Model file for the job. Use its own axes, mm. A direction names the side the tool comes from. Round coordinates to 2 decimals unless told otherwise and drop trailing zeros. Order: outer loops, then holes, each group sorted by start corner. A loop starts at its lowest first (then second) coordinate and runs counter-clockwise, first axis right, second up. Notation, with made-up numbers: (50, 7) -> (81, 7) arc R23 cw to (81, 24) -> close; hole circle Ø7 at (30, -34). An arc over 180 degrees is marked (long way). Put each result on its own line as item: value. Start each with the question number.
Q1. Probe L1, parallel to Y at x = -16.75, z = -68.5; L2, parallel to Z at x = -23.5, y = 28.6; L3, parallel to Z at x = -13.5, y = 23.5. List the from-to ranges inside material, lowest first.
Q2. Cut at C-C, the plane x = -27.25. List the corners of the cut face in (y, z), and give its area (3 significant figures).
Q3. Cut at D-D, the plane z = -9. List the corners of the cut face in (x, y).
Q4. Cut at A-A, the plane x = -6.5. List the corners of the cut face in (y, z).
Q5. Flat gauge pins, fed straight in: P1, Ø12, axis at y = 6.5, z = -33, coming from the -X side; P2, Ø6, axis at x = -23.5, z = -37.03, coming from the -Y side; P3, Ø10, axis at x = -25.5, y = 23, coming from the +Z side; P4, Ø9.5, axis at x = -11, z = -60, coming from the +Y side. Where does each tip first touch, or does it go through?
Q6. Cut at B-B, the plane y = 13. List the corners of the cut face in (x, z), and give its area (3 significant figures).
Q7. 3-axis set-ups, long thin cutter, end or side, ignore diameter. For faces 4 (the face through (-15.21, 14.676, -23.932)), 5 (the face through (-15, 0.76, -9)), 6 (the face through (-15, 0.76, -65)), 7 (the face through (-30, 13, -23)), 8 (the face through (-15, 29.174, -37)): which of +Z, -Z, +X, -X, +Y, -Y reach the whole face in a straight line?
Q8. Pull direction X, two halves, no side cores. Call faces 1 (the face through (-7.04, 28.8, -34.59)), 2 (the face through (0, 13, -23)), 3 (the face through (-14.79, 28.85, -46.8)): released by +X, released by -X, zero draft, split by the parting line, or undercut.
Autodesk Inventor part; units mm, degrees
ref_plane "YZ Plane" through (0, 0, 0) normal (1, 0, 0) x (0, 1, 0)
ref_plane "XZ Plane" through (0, 0, 0) normal (0, 1, 0) x (-1, 0, 0)
ref_plane "XY Plane" through (0, 0, 0) normal (0, 0, 1) x (1, 0, 0)
sketch "Boceto1" plane through (0, 0, 0) normal (0, 1, 0) x (-1, 0, 0)
  point P0 (0, 0)
sketch "Boceto2" plane through (0, 0, 0) normal (0, 1, 0) x (-1, 0, 0)
  line L0 (0, 0) -> (30, 0)
  line L1 (30, 0) -> (30, -20)
  line L2 (30, -20) -> (0, -20)
  line L3 (0, -20) -> (0, 0)
  dimension "d0" = 30
  dimension "d1" = 20
extrude "Placa1" add sketch "Boceto2" along normal blind 0.76
sketch "Boceto3" plane through (0, 0.1967, -19.2659) normal (0, -0.258819, -0.9659258) x (-1, 0, 0)
  line L0 (30, 0) -> (0, 0)
  line L1 (0, 0) -> (0, -30)
  line L2 (0, -30) -> (30, -30)
  line L3 (30, -30) -> (30, 0)
edge flange "Pestaña1" height 30 angle -75 thickness 0.76 bend radius 0.76 thickness toward (0, -0.258819, -0.9659258) relief tear relief width 0.76 relief depth 0.38 edges at (-15, 0, -20) wall of the first edge with corners at (-30, 0.1967, -19.2659) (0, 0.1967, -19.2659) (0, 29.1745, -27.0305) (-30, 29.1745, -27.0305)
bend "Doblez1"
corner "Esquina1"
sketch "Boceto4" plane through (-30, 28.4145, -27.0305) normal (0, 1, 0) x (-1, 0, 0)
  line L0 (-30, 0) -> (0, 0)
  line L1 (0, 0) -> (0, 20)
  line L2 (0, 20) -> (-30, 20)
  line L3 (-30, 20) -> (-30, 0)
edge flange "Pestaña2" height 20 angle -75 thickness 0.76 bend radius 0.76 thickness toward (0, 1, 0) relief tear relief width 0.76 relief depth 0.38 edges at (-15, 29.1745, -27.0305) wall of the first edge with corners at (0, 28.4145, -27.0305) (-30, 28.4145, -27.0305) (-30, 28.4145, -47.0305) (0, 28.4145, -47.0305)
bend "Doblez2"
corner "Esquina2"
sketch "Boceto5" plane through (-30, 28.9778, -46.2964) normal (0, 0.258819, -0.9659258) x (1, 0, 0)
  line L0 (30, 0) -> (0, 0)
  line L1 (0, 0) -> (0, -30)
  line L2 (0, -30) -> (30, -30)
  line L3 (30, -30) -> (30, 0)
edge flange "Pestaña3" height 30 angle -75 thickness 0.76 bend radius 0.76 thickness toward (0, 0.258819, -0.9659258) relief tear relief width 0.76 relief depth 0.38 edges at (-15, 29.1745, -47.0305) wall of the first edge with corners at (0, 28.9778, -46.2964) (-30, 28.9778, -46.2964) (-30, 0, -54.0609) (0, 0, -54.0609)
bend "Doblez3"
corner "Esquina3"
sketch "Boceto6" plane through (0, 0.76, -54.0609) normal (0, -1, 0) x (1, 0, 0)
  line L0 (-30, 0) -> (0, 0)
  line L1 (0, 0) -> (0, 20)
  line L2 (0, 20) -> (-30, 20)
  line L3 (-30, 20) -> (-30, 0)
edge flange "Pestaña4" height 20 angle -75 thickness 0.76 bend radius 0.76 thickness toward (0, -1, 0) relief tear relief width 0.76 relief depth 0.38 edges at (-15, 0, -54.0609) wall of the first edge with corners at (-30, 0.76, -54.0609) (0, 0.76, -54.0609) (0, 0.76, -74.0609) (-30, 0.76, -74.0609)
bend "Doblez4"
corner "Esquina4"
sketch "Boceto7" plane through (-30, 29.1745, -28.1968) normal (0, 1, 0) x (1, 0, 0)
  circle A0 centre (6.5, 8.8337) radius 2.5
  circle A1 centre (23.5, 8.8337) radius 2.5
  line L0 (0, 0) -> (0, 17.6673)
  line L1 (30, 0) -> (30, 17.6673)
  point P0 (30, -28.1968)
  dimension "d43" = 5
  dimension "d44" = 5
  dimension "d45" = 6.5
  dimension "d46" = 6.5
extrude "Extrusión1" cut sketch "Boceto7" against normal through all
equation "\"d46\" = d45"
equation "\"d2\" = Grosor"
equation "\"d3\" = Anchura_desahogo_plegado"
equation "\"d4\" = Profundidad_desahogo_plegado"
equation "\"d5\" = Remanente_mínimo"
equation "\"d6\" = Radiodetransición"
equation "\"d9\" = Radio_pliegue"
equation "\"d10\" = Tamaño_destalonado"
equation "\"d11\" = TamañoSeparación"
equation "\"d12\" = Tamaño_de_radio_de_Jacobi"
equation "\"d13\" = Anchura_desahogo_plegado"
equation "\"d14\" = Profundidad_desahogo_plegado"
equation "\"d15\" = Remanente_mínimo"
equation "\"d16\" = Radiodetransición"
equation "\"d19\" = Radio_pliegue"
equation "\"d20\" = Tamaño_destalonado"
equation "\"d21\" = TamañoSeparación"
equation "\"d22\" = Tamaño_de_radio_de_Jacobi"
equation "\"d23\" = Anchura_desahogo_plegado"
equation "\"d24\" = Profundidad_desahogo_plegado"
equation "\"d25\" = Remanente_mínimo"
equation "\"d26\" = Radiodetransición"
equation "\"d29\" = Radio_pliegue"
equation "\"d30\" = Tamaño_destalonado"
equation "\"d31\" = TamañoSeparación"
equation "\"d32\" = Tamaño_de_radio_de_Jacobi"
equation "\"d33\" = Anchura_desahogo_plegado"
equation "\"d34\" = Profundidad_desahogo_plegado"
equation "\"d35\" = Remanente_mínimo"
equation "\"d36\" = Radiodetransición"
equation "\"d39\" = Radio_pliegue"
equation "\"d40\" = Tamaño_destalonado"
equation "\"d41\" = TamañoSeparación"
equation "\"d42\" = Tamaño_de_radio_de_Jacobi"
equation "\"Radio_pliegue\" = Grosor"
equation "\"Anchura_desahogo_plegado\" = Grosor"
equation "\"Profundidad_desahogo_plegado\" = 0.5 * Grosor"
equation "\"Tamaño_destalonado\" = 4 * Grosor"
equation "\"Remanente_mínimo\" = 2 * Grosor"
equation "\"Radiodetransición\" = Radio_pliegue"
equation "\"Tamaño_de_radio_de_Jacobi\" = Radio_pliegue"
equation "\"TamañoSeparación\" = Grosor"
properties part number "placa tierra" material "Acero AISI 1006 85 LC"
Ans:
1. L1: y = 0 to 0.76
1. L2: z = -47.05 to -39.53, -34.53 to -27.01
1. L3: z = -48.55 to -47.76, -26.3 to -25.51
2. outline: (0, -74.06) -> (0.76, -74.06) -> (0.76, -55.23) arc R0.76 cw to (1.32, -54.49) -> (28.05, -47.33) arc R1.52 ccw to (29.17, -45.86) -> (29.17, -28.2) arc R1.52 ccw to (28.05, -26.73) -> (1.32, -19.57) arc R0.76 cw to (0.76, -18.83) -> (0.76, 0) -> (0, 0) -> (0, -18.83) arc R1.52 ccw to (1.13, -20.3) -> (27.85, -27.46) arc R0.76 cw to (28.41, -28.2) -> (28.41, -45.86) arc R0.76 cw to (27.85, -46.6) -> (1.13, -53.76) arc R1.52 ccw to (0, -55.23) -> close
2. area: 88.6 mm^2
3. outline: (-30, 0) -> (0, 0) -> (0, 0.76) -> (-30, 0.76) -> close
4. outline: (0, -74.06) -> (0.76, -74.06) -> (0.76, -55.23) arc R0.76 cw to (1.32, -54.49) -> (28.05, -47.33) arc R1.52 ccw to (29.17, -45.86) -> (29.17, -39.53) -> (28.41, -39.53) -> (28.41, -45.86) arc R0.76 cw to (27.85, -46.6) -> (1.13, -53.76) arc R1.52 ccw to (0, -55.23) -> close; (0, -18.83) arc R1.52 ccw to (1.13, -20.3) -> (27.85, -27.46) arc R0.76 cw to (28.41, -28.2) -> (28.41, -34.53) -> (29.17, -34.53) -> (29.17, -28.2) arc R1.52 ccw to (28.05, -26.73) -> (1.32, -19.57) arc R0.76 cw to (0.76, -18.83) -> (0.76, 0) -> (0, 0) -> close
5. P1: passes through
5. P2: stops at y = 28.41
5. P3: stops at z = -24.04
5. P4: stops at y = 0.76
6. outline: (-30, -51.36) -> (0, -51.36) -> (0, -50.58) -> (-30, -50.58) -> close; (-30, -23.48) -> (0, -23.48) -> (0, -22.7) -> (-30, -22.7) -> close
6. area: 47.2 mm^2
7. face 4: +X, -X, -Y
7. face 5: +Z, +X, -X, +Y
7. face 6: -Z, +X, -X, +Y
7. face 7: +Z, -Z, -X, +Y, -Y
7. face 8: +Z, -Z, +X, -X, +Y
8. face 1: undercut
8. face 2: released by +X
8. face 3: zero draft
